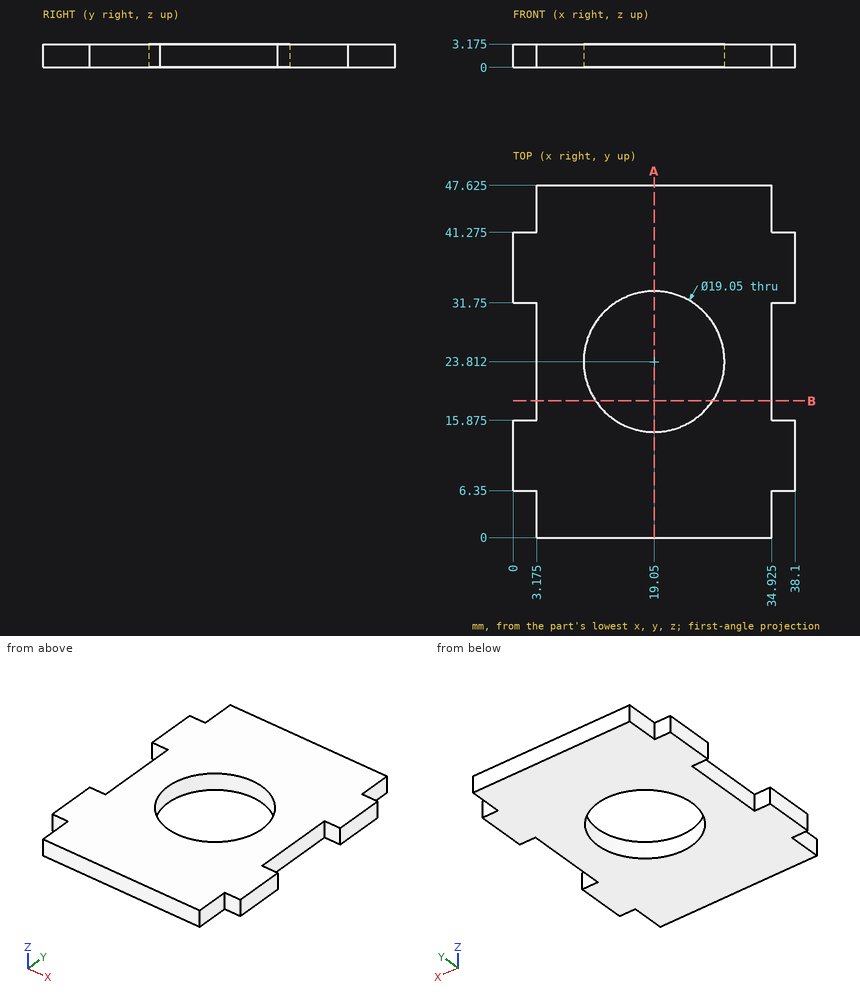
Can you work these out from the drawing? Everything is in mm from the part's minimum corner. Coordinates: 2 decimals unless noted, no trailing zeros. Loops run counter-clockwise (first coordinate to the right, second up) from the corner with the lowest first, then second, coordinate; pieces in that order, holes last.
1. I need wall thicknesses on L1, parallel to X at y = 23.5, z = 2.5 (1 decimal); L2, parallel to Y at x = 19.05, z = 1 (1 decimal); L3, parallel to X at y = 32, z = 0.2 (1 decimal). Which ranges of each line are inside material? Lowest first, please.
2. Imagine slicing it at B-B, the plane y = 18.5. Please give me the cut outline in (x, z) (1 decimal).
3. Imagine slicing it at A-A, the plane x = 19.05. Please give me the cut outline in (y, z) (1 decimal).
4. For P1, Ø1, axis at x = 36, z = 2.5, coming from the +Y side (1 decimal); P2, Ø1, axis at x = 37, z = 1, coming from the -Y side; P3, Ø1, axis at y = 5, z = 2.5, coming from the +X side (1 decimal), each with a flat end and sliding along its axis, tell me the tip position at first contact or that it passes through.
Taken from the geometry:
1. L1: x = 3.2 to 9.5, 28.6 to 34.9
1. L2: y = 0 to 14.3, 33.3 to 47.6
1. L3: x = 0 to 14.2, 23.9 to 38.1
2. outline: (3.2, 0) - (11.1, 0) - (11.1, 3.2) - (3.2, 3.2) - close; (27, 0) - (34.9, 0) - (34.9, 3.2) - (27, 3.2) - close
3. outline: (0, 0) - (14.3, 0) - (14.3, 3.2) - (0, 3.2) - close; (33.3, 0) - (47.6, 0) - (47.6, 3.2) - (33.3, 3.2) - close
4. P1: stops at y = 41.3
4. P2: stops at y = 6.35
4. P3: stops at x = 34.9
